Verification items for the finished model (mm, model axes). Give positions to 0.01 mm unless a question says otherwise; leave off trailing zeros. Order: outer loops, then holes, each group sorted by start corner. A loop starts at its lowest first (then second) coordinate and runs counter-clockwise, first axis right, second up. Notation, with made-up numbers: (2.25, -9) -> (23.25, -9) arc R27 ccw to (23.25, 17) -> close; hole circle Ø9 at (61.5, -4). An arc over 180 degrees is marked (long way). Return JSON: item names as keys, results as strings. Group by question number.
(1) Release check for a two-part mould opening along X. For faces 1 (the face through (1, 0, 14)), 2 (the face through (17.87, 1.52, -18.05)), 3 (the face through (-28.144, 1.478, 50.613)) record: pulls with the +X half, pulls with the -X half, needs draft (parallel to the pull), parting line crosses it, or undercut.
(2) Cross-section at D-D on z = 42.5. Enter the section's corners in (x, y).
(3) Thickness scan on line 1 along X through (y, z) = (0.4, 142.5) (3 decimals); line 2 along X through (y, z) = (2.8, 63); line 3 along Z through (x, y) = (-36.5, 2.3). Record the ranges inside material, lowest first.
(4) Cross-section at C-C on z = 0. Enter the section's corners in (x, y), then the cut area to 3 significant figures.
(5) Cross-section at A-A on z = 82.5. Enter the section's corners in (x, y) (3 decimals), then the cut area to 3 significant figures.
(6) Depth check by flat-ended pin: pin 1 Ø0.9 at (y, z) = (1, 121) entering from -X; pin 2 Ø1.5 at (x, y) = (-34, 1.5) entering from -Z; pin 3 Ø1 at (y, z) = (0.5, -3.5) entering from +X. Enter the tip coordinate at first touch or a pass-through.
from build123d import *

# Parameters (mm, degrees)
BOSS_EXTRUDE1_DEPTH = 2.9972
SKETCH2_R           = 7.62
CUT_EXTRUDE1_DEPTH  = 197.198393122
CUT_EXTRUDE2_DEPTH  = 197.198393122
SKETCH4_R           = 20.32
CUT_EXTRUDE3_DEPTH  = 197.198393122
CUT_EXTRUDE4_DEPTH  = 197.198393122
SKETCH6_W           = 3.556
SKETCH6_H           = 9.751681081
CUT_EXTRUDE5_DEPTH  = 197.198393122


with BuildPart() as part:
    # Sketch1 → Boss-Extrude1 (new body)
    with BuildSketch(Plane(origin=(0, 0, 0), x_dir=(1, 0, 0), z_dir=(0, 1, 0))):
        with BuildLine():
            Line((12.7, -75.184), (12.7, -176.784))
            ThreePointArc((12.7, -176.784), (0, -189.484), (-12.7, -176.784))
            Line((-12.7, -176.784), (-12.7, -75.184))
            Line((-12.7, -75.184), (-44.026400327, -25.343955378))
            ThreePointArc((-44.026400327, -25.343955378), (0, 50.8), (44.026400327, -25.343955378))
            Line((44.026400327, -25.343955378), (12.7, -75.184))
        make_face()
    extrude(amount=BOSS_EXTRUDE1_DEPTH)

    # Sketch2 → Cut-Extrude1 (cut, through all)
    with BuildSketch(Plane(origin=(0, 2.9972, 0), x_dir=(1, 0, 0), z_dir=(0, 1, 0))):
        with Locations(Location((-33.02, 0, 0), (0, 0, 270))):
            Circle(SKETCH2_R)
        with Locations(Location((-23.348665915, 23.348665915, 0), (0, 0, 270))):
            Circle(SKETCH2_R)
        with Locations(Location((0, 33.02, 0), (0, 0, 270))):
            Circle(SKETCH2_R)
        with Locations(Location((23.348665915, 23.348665915, 0), (0, 0, 270))):
            Circle(SKETCH2_R)
        with Locations(Location((33.02, 0, 0), (0, 0, 270))):
            Circle(SKETCH2_R)
    extrude(amount=-CUT_EXTRUDE1_DEPTH, mode=Mode.SUBTRACT)

    # Sketch3 → Cut-Extrude2 (cut, through all)
    with BuildSketch(Plane(origin=(0, 2.9972, 0), x_dir=(1, 0, 0), z_dir=(0, 1, 0))):
        with BuildLine():
            Line((-15.316948027, -30.962542518), (-1.255828352, -30.962542518))
            ThreePointArc((-1.255828352, -30.962542518), (-21.463230594, 22.351417773), (30.988, 0))
            Line((30.988, 0), (34.544, 0))
            ThreePointArc((34.544, 0), (-18.223326856, 29.346180234), (-15.316948027, -30.962542518))
        make_face()
    extrude(amount=-CUT_EXTRUDE2_DEPTH, mode=Mode.SUBTRACT)

    # Sketch4 → Cut-Extrude3 (cut, through all)
    with BuildSketch(Plane(origin=(0, 2.9972, 0), x_dir=(1, 0, 0), z_dir=(0, 1, 0))):
        with Locations((0, -39.624)):
            Circle(SKETCH4_R)
    extrude(amount=-CUT_EXTRUDE3_DEPTH, mode=Mode.SUBTRACT)

    # Sketch5 → Cut-Extrude4 (cut, through all)
    with BuildSketch(Plane(origin=(0, 2.9972, 0), x_dir=(1, 0, 0), z_dir=(0, 1, 0))):
        with BuildLine():
            Line((6.985, -72.009), (6.985, -173.609))
            ThreePointArc((6.985, -173.609), (0, -180.594), (-6.985, -173.609))
            Line((-6.985, -173.609), (-6.985, -72.009))
            ThreePointArc((-6.985, -72.009), (0, -65.024), (6.985, -72.009))
        make_face()
    extrude(amount=-CUT_EXTRUDE4_DEPTH, mode=Mode.SUBTRACT)

    # Sketch6 → Cut-Extrude5 (cut, through all)
    with BuildSketch(Plane(origin=(0, 2.9972, 0), x_dir=(1, 0, 0), z_dir=(0, 1, 0))):
        with Locations((0.254, -62.435855584)):
            Rectangle(SKETCH6_W, SKETCH6_H)
    extrude(amount=-CUT_EXTRUDE5_DEPTH, mode=Mode.SUBTRACT)


solid = part.part
Verdict:
{
 "1": {"face 1": "needs draft", "face 2": "undercut", "face 3": "pulls with the -X half"},
 "2": {"outline": "(-33.24, 0) -> (-20.12, 0) -> (-20.12, 3) -> (-33.24, 3) -> close; (20.12, 0) -> (33.24, 0) -> (33.24, 3) -> (20.12, 3) -> close"},
 "3": {"line 1": "-12.7 to -6.985, 6.985 to 12.7", "line 2": "-20.36 to -1.52, 2.03 to 20.36", "line 3": "-35.33 to -6.78, 6.78 to 37.32"},
 "4": {"outline": "(-50.8, 0) -> (-40.64, 0) -> (-40.64, 3) -> (-50.8, 3) -> close; (-25.4, 0) -> (25.4, 0) -> (25.4, 3) -> (-25.4, 3) -> close; (40.64, 0) -> (50.8, 0) -> (50.8, 3) -> (40.64, 3) -> close", "area": "213 mm²"},
 "5": {"outline": "(-12.7, 0) -> (-6.985, 0) -> (-6.985, 2.997) -> (-12.7, 2.997) -> close; (6.985, 0) -> (12.7, 0) -> (12.7, 2.997) -> (6.985, 2.997) -> close", "area": "34.3 mm²"},
 "6": {"pin 1": "x = -12.7", "pin 2": "z = -38.41", "pin 3": "x = 50.71"}
}
